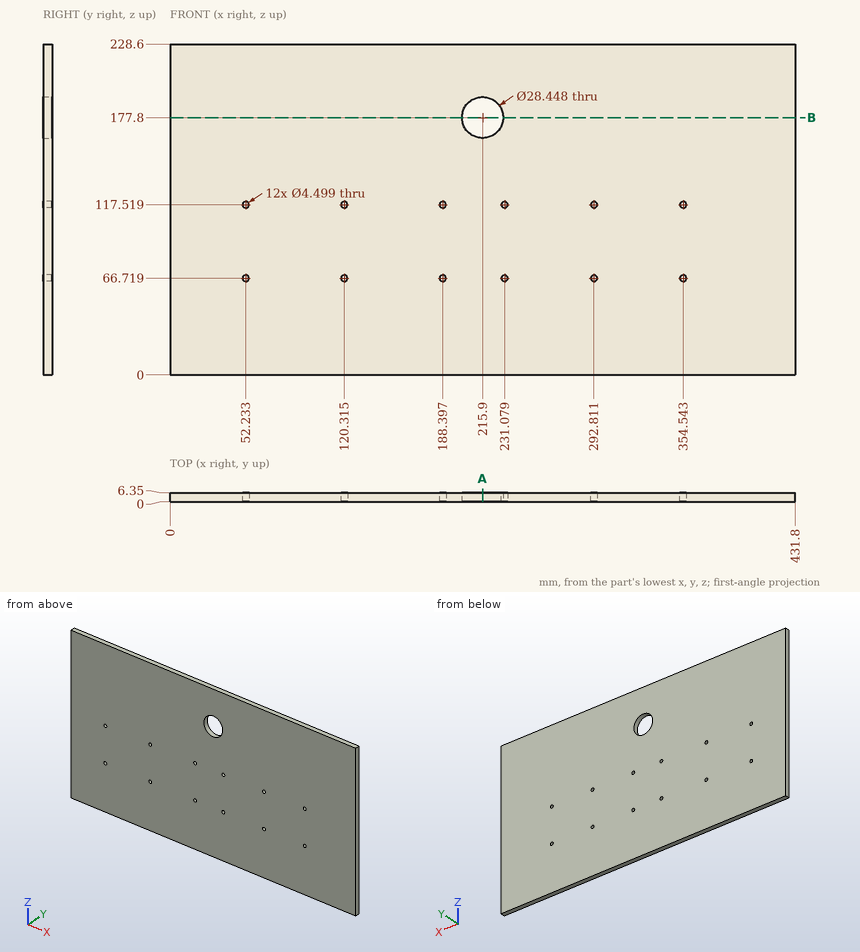
Input: dimensioned drawing with shaded views. Units: mm. Origin: part minimum x, y, z. Round coordinates to 2 decimals unless told otherwise and drop trailing zeros. Order: outer loops, then holes, each group sorted by start corner. A loop starts at its lowest first (then second) coordinate and runs counter-clockwise, first axis right, second up. Notation, with made-up numbers: (-13.75, 30.5) - (-6.75, 30.5) arc R11 cw to (-6.75, 48.5) - close; hole circle Ø5 at (-12, -30.75). An arc over 180 degrees is marked (long way). Use CSV: the item, a comma, the result in double quotes. Start each with the question number.
Q1. Section query B-B (z = 177.8). Return loops of the section in (x, y), and give its area (3 significant figures).
Q2. Material intervals for line 1 along Z through (x, y) = (54, 6) (1 decimal); line 2 along Z through (x, y) = (291.5, 2.75); line 3 along Z through (x, y) = (214, 6.25), sorted ascending. Write a range as from..to.
Q3. Section query A-A (x = 215.9). Return loops of the section in (y, z).
Q4. First-contact query: pin 1 (6 mm diameter, centred on x = 292.81, z = 117.52, fed in from -Y); pin 2 (4 mm diameter, centred on x = 188.4, z = 117.52, fed in from +Y). Flat tips, straight axial feed; report the tip coordinate or a pass-through.
Result set:
1,outline,"(0, 0) - (201.68, 0) - (201.68, 6.35) - (0, 6.35) - close; (230.12, 0) - (431.8, 0) - (431.8, 6.35) - (230.12, 6.35) - close"
1,area,"2,560 mm2"
2,line 1,"z = 0..65.3, 68.1..116.1, 118.9..228.6"
2,line 2,"z = 0..64.89, 68.55..115.69, 119.35..228.6"
2,line 3,"z = 0..163.7, 191.9..228.6"
3,outline,"(0, 0) - (6.35, 0) - (6.35, 163.58) - (0, 163.58) - close; (0, 192.02) - (6.35, 192.02) - (6.35, 228.6) - (0, 228.6) - close"
4,pin 1,"stops at y = 0"
4,pin 2,"passes through"
